Build history of the part. All positions in model axes, mm. Coordinates: 2 decimals unless noted, no trailing zeros. Order: outer loops, then holes, each group sorted by start corner. A loop starts at its lowest first (then second) coordinate and runs counter-clockwise, first axis right, second up. Notation, with made-up numbers: (61, 61.25) - (99, 61.25) arc R13 cw to (99, 71.25) - close; hole circle Ø10 at (31, 10.5). An arc over 180 degrees is marked (long way). Return JSON: item names as keys, results as strings.
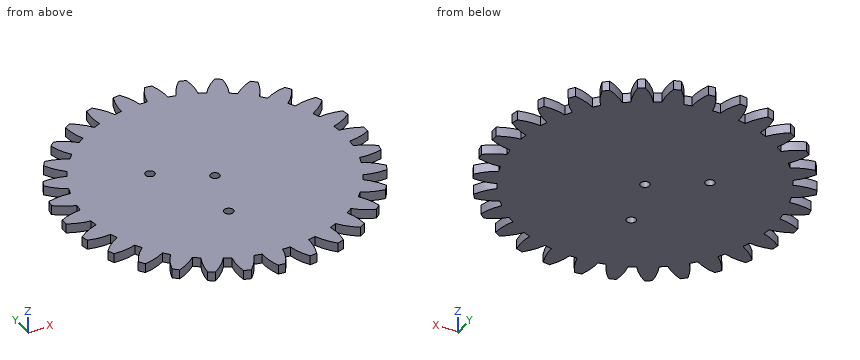
from build123d import *

# Parameters (mm, degrees)
SKETCH1_R           = 48
BOSS_EXTRUDE1_DEPTH = 3
CUT_EXTRUDE1_DEPTH  = 68.948509917
CIRPATTERN1_COUNT   = 30
SKETCH7_R           = 1.47
CUT_EXTRUDE2_DEPTH  = 68.835567074
SKETCH8_R           = 1.47
CUT_EXTRUDE3_DEPTH  = 68.835567074


with BuildPart() as part:
    # Sketch1 → Boss-Extrude1 (new body)
    with BuildSketch(Plane.XY):
        Circle(SKETCH1_R)
    extrude(amount=BOSS_EXTRUDE1_DEPTH)

    # Sketch2 → Cut-Extrude1 (cut, through all)
    with BuildSketch(Plane.XY.offset(3)):
        with BuildLine():
            ThreePointArc((-1.20388032, 41.232428648), (0, 41.25), (1.20388032, 41.232428648))
            ThreePointArc((1.20388032, 41.232428648), (2.228958391, 44.672086233), (3.916100076, 47.839984952))
            ThreePointArc((3.916100076, 47.839984952), (0, 48), (-3.916100076, 47.839984952))
            ThreePointArc((-3.916100076, 47.839984952), (-2.228958391, 44.672086233), (-1.20388032, 41.232428648))
        make_face()
    cut_extrude1 = extrude(amount=-CUT_EXTRUDE1_DEPTH, mode=Mode.SUBTRACT)

    # CirPattern1: Cut-Extrude1 ×30 about axis
    cirpattern1_axis = Axis((0, 0, 0), (0, 0, 1))
    for i in range(1, CIRPATTERN1_COUNT):
        add(cut_extrude1.rotate(cirpattern1_axis, i * 360 / CIRPATTERN1_COUNT), mode=Mode.SUBTRACT)

    # Sketch7 → Cut-Extrude2 (cut, through all)
    with BuildSketch(Plane(origin=(0, 0, 0), x_dir=(-1, 0, 0), z_dir=(0, 0, -1))):
        Circle(SKETCH7_R)
    extrude(amount=-CUT_EXTRUDE2_DEPTH, mode=Mode.SUBTRACT)

    # Sketch8 → Cut-Extrude3 (cut, through all)
    with BuildSketch(Plane(origin=(0, 0, 0), x_dir=(-1, 0, 0), z_dir=(0, 0, -1))):
        with Locations((5.200050154, -17.363038426)):
            Circle(SKETCH8_R)
        with Locations((15.425535223, 9.516747768)):
            Circle(SKETCH8_R)
    extrude(amount=-CUT_EXTRUDE3_DEPTH, mode=Mode.SUBTRACT)


solid = part.part
1. Cut at C-C on z = 2. State how many separate pieces and enclosed holes the cut face has, plus the area to 3 significant figures.
Check values:
{"separate pieces": "1", "enclosed holes": "3", "area": "6,280 mm²"}
2. Cut at B-B on x = 0. Give the cut face in (y, z), plus the area to 3 significant figures.
Check values:
{"outline": "(-41.25, 0) - (-1.47, 0) - (-1.47, 3) - (-41.25, 3) - close; (1.47, 0) - (41.25, 0) - (41.25, 3) - (1.47, 3) - close", "area": "239 mm²"}
3. Probe L1, parallel to Y at x = 0, z = 0.8; L2, parallel to X at y = -28, z = 2.65; L3, parallel to Y at x = -35.5, z = 0.7. List the from-to ranges inside material, lowest first.
Check values:
{"L1": "-41.25 to -1.47, 1.47 to 41.25", "L2": "-38.99 to -34.07, -30.29 to 30.29, 34.07 to 38.99", "L3": "-28.5 to -22.01, -21.01 to 21.01, 22.01 to 28.5"}
4. Cut at A-A on y = 0. Give the cut face in (x, z), plus the area to 3 significant figures.
Check values:
{"outline": "(-48, 0) - (-1.47, 0) - (-1.47, 3) - (-48, 3) - close; (1.47, 0) - (48, 0) - (48, 3) - (1.47, 3) - close", "area": "279 mm²"}
5. Drop flat-ended pins along their axis: pin 1 (2.5 mm diameter, centred on x = 0, y = 0, fed in from -Z); pin 2 (1.5 mm diameter, centred on y = -34, z = 1, fed in from -X). Give the stop position or say it passes through.
Check values:
{"pin 1": "through", "pin 2": "x = -32.89"}
6. Cut at D-D on x = -27. Give the cut face in (y, z).
Check values:
{"outline": "(-34.12, 0) - (34.12, 0) - (34.12, 3) - (-34.12, 3) - close"}
